For this review, take the finished solid that the model builds, in its own axes (mm). A direction names the side the tool comes from. Round coordinates to 2 decimals unless told otherwise and drop trailing zeros. Order: outer loops, then holes, each group sorted by start corner. A loop starts at its lowest first (then second) coordinate and runs counter-clockwise, first axis right, second up. Notation, with made-up numbers: M -37,25.25 L -20,25.25 A20 cw -20,44.25 Z; hole C 79.5,41.5 d1. An arc over 180 degrees is marked long. Put each result on its own line as item: value.
Autodesk Inventor part; units mm, degrees
ref_plane "YZ Plane" through (0, 0, 0) normal (1, 0, 0) x (0, 1, 0)
ref_plane "XZ Plane" through (0, 0, 0) normal (0, 1, 0) x (-1, 0, 0)
ref_plane "XY Plane" through (0, 0, 0) normal (0, 0, 1) x (1, 0, 0)
sketch "Sketch1" plane through (0, 0, 0) normal (0, 0, 1) x (1, 0, 0)
  arc A0 (-18.5, 0) -> (18.5, 0) centre (0, 0) ccw
  line L0 (18.5, 0) -> (32.0244, 0)
  line L1 (96, -23) -> (-64, -23)
  circle A1 centre (24, -7) radius 1.85
  circle A2 centre (-24, -7) radius 1.85
  line L2 (32, -20) -> (32, 6)
  line L3 (-32, 6) -> (-32, -20)
  line L4 (-18.5, 0) -> (-32, 0)
  line L5 (-32, -20) -> (-32, -23)
  arc A3 (29, -23) -> (32, -20) centre (29, -20) ccw
  arc A4 (-32, -20) -> (-29, -23) centre (-29, -20) ccw
  point P0 (32, 0)
extrude "Extrusion1" add sketch "Sketch1" along normal blind 16 contours A0 L0 L2 A3 L1 A4 L3 L4
sketch "Sketch2" plane through (-29, -23, 0) normal (0, -1, 0) x (1, 0, 0)
  circle A0 centre (45, 10) radius 1.85
  circle A1 centre (13, 10) radius 1.85
  point P0 (29, 0)
hole "Hole1" at (16, -23, 10) at (-16, -23, 10) direction (0, 1, 0) diameter 2.7051 end through all
fillet "Fillet1" radius 2 4 edges at (32, 0, 8) (18.5, 0, 8) (-18.5, 0, 8) (-32, 0, 8)
properties part number "motorsupport"
(1) To check wall thickness, follow L1, parallel to X at y = -19.25, z = 10; L2, parallel to X at y = -12, z = 9.5; L3, parallel to Z at x = 16, y = -17. State the ranges of each line that lie inside material, in increasing order.
A:
L1: x = -32 to -17.35, -14.65 to 14.65, 17.35 to 32
L2: x = -32 to -17.26, -14.74 to -14.08, 14.08 to 14.74, 17.26 to 32
L3: z = 0 to 8.65, 11.35 to 16
(2) Add section C-C on z = 3.25. Give the boundary of the cut face in (x, y).
A:
outline: M -32,-20 A3 ccw -29,-23 L 29,-23 A3 ccw 32,-20 L 32,-2 A2 ccw 30,0 L 20.4,0 A2 ccw 18.41,-1.8 A18.5 cw -18.41,-1.8 A2 ccw -20.4,0 L -30,0 A2 ccw -32,-2 Z; hole C -24,-7 d3.7; hole C 24,-7 d3.7
(3) Draft analysis for pull direction X (two halves, no side actions). For faces 3 (the face through (0, -19, 0)), 4 (the face through (-17.34, -16.43, 10.18)), 5 (the face through (-19.044, -0.532, 8.112)), 6 (the face through (31.43, -0.6, 8.11)), state which applies: released by +X, released by -X, zero draft, split by the parting line, or undercut.
A:
face 3: zero draft
face 4: undercut
face 5: undercut
face 6: released by +X
(4) Add section A-A on x = 24. Give the boundary of the cut face in (y, z), then the cut area to 3 significant figures.
A:
outline: M -23,0 L -8.85,0 L -8.85,16 L -23,16 Z; M -5.15,0 L 0,0 L 0,16 L -5.15,16 Z
area: 309 mm2
(5) Add section D-D on y = -16.5. Give the boundary of the cut face in (x, z), then the cut area to 3 significant figures.
A:
outline: M -32,0 L -8.37,0 L -8.37,16 L -32,16 Z; M 8.37,0 L 32,0 L 32,16 L 8.37,16 Z; hole C -16,10 d2.71; hole C 16,10 d2.71
area: 745 mm2
(6) For faces 1 (the face through (25, 0, 8)), 2 (the face through (19.074, -0.505, 8.112)), list the 3-axis set-ups (+Z, -Z, +X, -X, +Y, -Y) from which the entire face can be reached by the end or side of a thin tool; tool diameter is ignored.
A:
face 1: +Z, -Z, +X, -X, +Y
face 2: +Z, -Z, +Y
(7) Add section B-B on y = -10. Give the boundary of the cut face in (x, z).
A:
outline: M -32,0 L -15.56,0 L -15.56,8.72 A1.35 cw long -15.56,11.28 L -15.56,16 L -32,16 Z; M 15.56,0 L 32,0 L 32,16 L 15.56,16 L 15.56,11.28 A1.35 cw long 15.56,8.72 Z
